from build123d import *

# Parameters (mm, degrees)
F1_DEPTH = 7
F3_DEPTH = 40.4378042152
F4_DEPTH = 5.8827169768
F5_R     = 1.75
F6_DEPTH = 2


with BuildPart() as f1:
    # F0 (on Front) → F1 (new body)
    with BuildSketch(Plane.XZ):
        Polygon((27.5, 15), (27.5, 25), (-27.5, 25), (-27.5, -25), align=None)
    extrude(amount=F1_DEPTH)

    # F2 (on face) → F3 (cut, through all)
    with BuildSketch(Plane(origin=(2.3783783784, 0, -3.2702702703), x_dir=(0.8087360843, 0, 0.5881716977), z_dir=(0.5881716977, 0, -0.8087360843))):
        Polygon((31.0628177835, 7), (-36.9445347602, 7), (31.0628177835, 5.5), align=None)
        Polygon((31.0628177835, 1.5), (-36.9445347602, 0), (31.0628177835, 0), align=None)
    extrude(amount=-F3_DEPTH, mode=Mode.SUBTRACT)

    # F4 (cut, through all): faces of the model
    f4_faces = [f1.faces().sort_by_distance(p)[0] for p in [
        (23.8636363636, -6.25, 20),
        (23.8636363636, -0.75, 20),
    ]]
    extrude(f4_faces, amount=-F4_DEPTH, mode=Mode.SUBTRACT)

    # F5 (on face) → F6 (cut)
    with BuildSketch(Plane(origin=(-0.0145283595, -0.8144686369, -0.0105660796), x_dir=(-0.9998409705, 0.017832, 0.0002313341), z_dir=(0.0178335005, 0.9997568455, 0.0129698185))):
        with Locations((7.489843337, 10.0109374025)):
            Circle(F5_R)
    extrude(amount=-F6_DEPTH, mode=Mode.SUBTRACT)


solid = f1.part
The model under review builds one solid part; all positions refer to its coordinate system, in mm. A direction names the side the tool comes from. Give positions to 0.01 mm unless a question says otherwise; leave off trailing zeros. Loops run counter-clockwise (first coordinate to the right, second up) from the corner with the lowest first, then second, coordinate; pieces in that order, holes last. Notation, with made-up numbers: (88, -30.75) -> (93, -30.75) arc R20 cw to (93, 6.25) -> close; hole circle Ø11 at (67, -30). An arc over 180 degrees is marked (long way). Answer as a JSON object with one key per item and string values. Group by question number.
Q1. Insertion check: pin 1 (4 mm diameter, centred on x = -13.5, z = 10, fed in from -Y); pin 2 (3.5 mm diameter, centred on x = 23, z = 21, fed in from +Y); pin 3 (2 mm diameter, centred on y = -3.5, z = -19.5, fed in from +X). Each pin has a flat end and moves straight along its axis. Give the tip position at first contact, or say it passes through.
Q2. Wall thickness on line 1 along Z through (x, y) = (23, -5.25); line 2 along Y through (x, z) = (-4.5, 9); line 3 along Z through (x, y) = (-8, -5): over which ranges is each line inside the solid? List them lowest first.
Q3. Take a section at A-A (z = 19.5). Write out the cut boundary in (x, y).
Q4. Tool access review of faces 1 (the flat face through (27.5, -3, 20)), 2 (the flat face through (24, -5.5, 22)), 3 (the flat face through (24, -1.5, 22)): name each direction out of +Z, -Z, +X, -X, +Y, -Y from which nothing blocks a thin tool from reaching the whole face with its end or side.
Q5. Take a section at C-C (y = -3.75). Write out the cut boundary in (x, z), plus the area to 3 significant figures.
Q6. Draft analysis for pull direction Z (two halves, no side actions). For faces 4 (the cylindrical face through (-8.461, -1.799, 11.464)), 5 (the flat face through (-27.5, -3, 0)), 6 (the flat face through (0, -3, -5)), state which applies: pulls with the +Z half, pulls with the -Z half, needs draft (parallel to the pull), parting line crosses it, or undercut.
Q7. Take a section at B-B (x = 1). Write out the cut boundary in (y, z), plus the area to 3 significant figures.
Answer below:
{
 "1": {"pin 1": "stops at y = -6.34", "pin 2": "stops at y = -1.46", "pin 3": "stops at x = -18.56"},
 "2": {"line 1": "z = 11.73 to 25", "line 2": "y = -6.15 to -0.85", "line 3": "z = -10.82 to 25"},
 "3": {"outline": "(-27.5, -6.42) -> (24.23, -5.5) -> (27.5, -5.5) -> (27.5, -1.5) -> (24.23, -1.5) -> (-27.5, -0.58) -> close"},
 "4": {"face 1": "+Z, -Z, +X, +Y, -Y", "face 2": "+Z, +X, -Y", "face 3": "+Z, +X, +Y"},
 "5": {"outline": "(-27.5, -25) -> (27.5, 15) -> (27.5, 25) -> (-27.5, 25) -> close", "area": "1,650 mm2"},
 "6": {"face 4": "undercut", "face 5": "needs draft", "face 6": "pulls with the -Z half"},
 "7": {"outline": "(-6.22, -4.27) -> (-0.78, -4.27) -> (-1.16, 25) -> (-5.84, 25) -> close", "area": "148 mm2"}
}
